Geometry: see drawing. Coordinates: mm, zero at the bounding-box minimum. A direction names the side the tool comes from. Give positions to 0.01 mm unless a question says otherwise; leave off trailing zeros. Write each loop counter-clockwise with the first axis right and the second up, starting at its lowest first coordinate (ties: lowest second). Pieces come first, ordered by that corner, then holes. Notation, with made-up numbers: (9.25, 66) - (15.25, 66) arc R20 cw to (15.25, 83) - close; hole circle Ø2 at (78, 67.5). An arc over 180 degrees is marked (long way). Return JSON: item names as keys, results as strings.
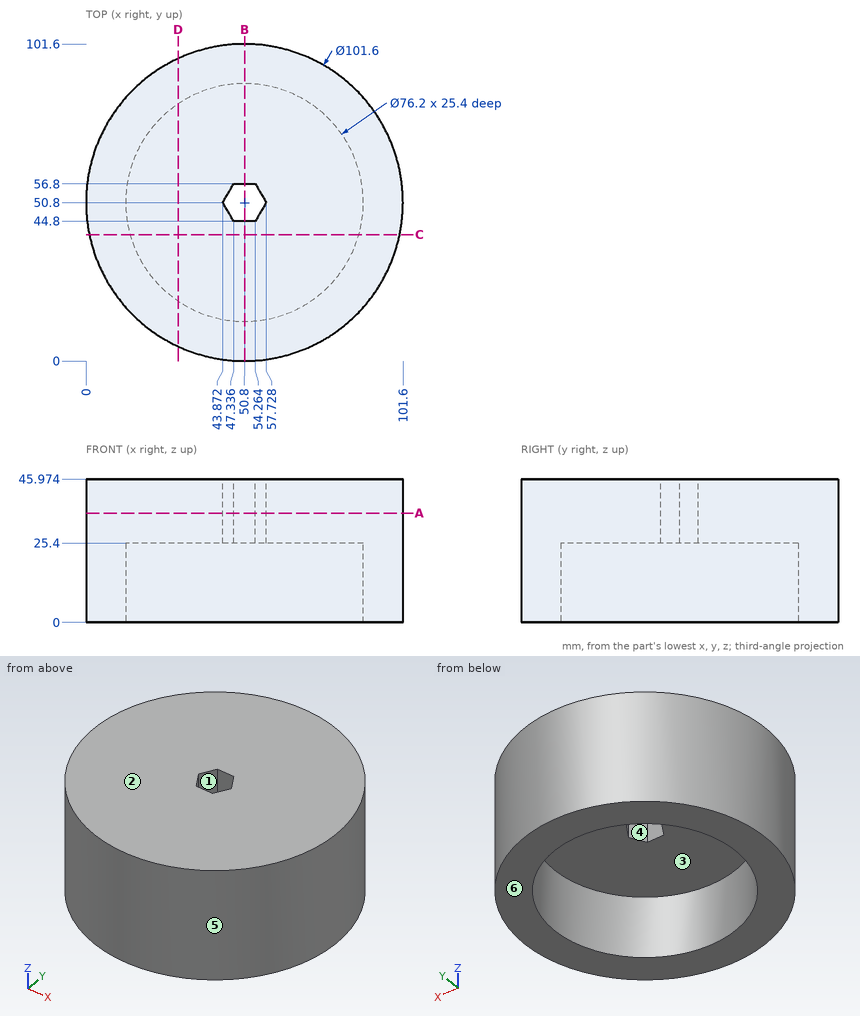
Q1. Material intervals for probe 1 along Y at (x, z) = (50, 11); probe 2 along Z at (x, y) = (79, 35); probe 3 along X at (y, z) = (56, 3), sorted ascending. Write a range as [from, to].
Answer key:
{"probe 1": "y = [0.01, 12.71], [88.89, 101.59]", "probe 2": "z = [25.4, 45.97]", "probe 3": "x = [0.27, 13.06], [88.54, 101.33]"}
Q2. Mould query, pull axis Y, two halves, no side actions, for the marked faces 4, 5 and 6. Classes: pulls with the +Y half, pulls with the -Y half, needs draft (parallel to the pull), parting line crosses it, or undercut.
Answer key:
{"face 4": "undercut", "face 5": "parting line crosses it", "face 6": "needs draft"}
Q3. Section query B-B, the plane x = 50.8. Return the cut outline in (y, z), plus the area to 3 significant figures.
Answer key:
{"outline": "(0, 0) - (12.7, 0) - (12.7, 25.4) - (44.8, 25.4) - (44.8, 45.97) - (0, 45.97) - close; (56.8, 25.4) - (88.9, 25.4) - (88.9, 0) - (101.6, 0) - (101.6, 45.97) - (56.8, 45.97) - close", "area": "2,490 mm^2"}
Q4. Section query D-D, the plane x = 29.5. Return the cut outline in (y, z), plus the area to 3 significant figures.
Answer key:
{"outline": "(4.68, 0) - (19.21, 0) - (19.21, 25.4) - (82.39, 25.4) - (82.39, 0) - (96.92, 0) - (96.92, 45.97) - (4.68, 45.97) - close", "area": "2,640 mm^2"}
Q5. Pin query (flat end, axial travel): P1, Ø8, axis at x = 90, z = 16, coming from the -Y side; P2, Ø8, axis at x = 85.5, z = 9, coming from the +Y side; P3, Ø1.5, axis at x = 74.5, z = 14.5, coming from the +Y side. Return the tip coordinate at first contact, or that it passes through.
Answer key:
{"P1": "stops at y = 14.17", "P2": "stops at y = 91.27", "P3": "stops at y = 96.12"}
Q6. Section query C-C, the plane y = 40.5. Return the cut outline in (x, z) (1 decimal).
Answer key:
{"outline": "(1.1, 0) - (14.1, 0) - (14.1, 25.4) - (87.5, 25.4) - (87.5, 0) - (100.5, 0) - (100.5, 46) - (1.1, 46) - close"}
Q7. Section query A-A, the plane z = 35. Return the cut outline in (x, y).
Answer key:
{"outline": "circle Ø101.6 at (50.8, 50.8); hole (43.87, 50.8) - (47.34, 44.8) - (54.26, 44.8) - (57.73, 50.8) - (54.26, 56.8) - (47.34, 56.8) - close"}
Q8. Set-up query: the marked faces 1, 2 and 3. Return all of +Z, -Z, +X, -X, +Y, -Y with unobstructed straight access to the full face (end or side cutting, diameter ignored); none if empty.
Answer key:
{"face 1": "+Z, -Z", "face 2": "+Z, +X, -X, +Y, -Y", "face 3": "-Z"}
